```python
from build123d import *

# Parameters (mm, degrees)
CHAMFER1_SIZE          = 0.5
TROU_TARAUD_M30_REACH  = 42.606
TROU_TARAUD_M30_BORE_R = 1.25
CIRPATTERN1_COUNT      = 2
CIRPATTERN1_ANGLE      = 90


with BuildPart() as part:
    # Sketch1 → Revolve1 (revolve)
    with BuildSketch(Plane.XY, mode=Mode.PRIVATE) as revolve1_sk:
        Polygon((-7.15, 4), (-7.15, 14.67), (-6.65, 14.67), (-7.15, 19), (-6.15, 19), (-5, 16.17), (5, 16.17), (6.15, 19), (7.15, 19), (6.65, 14.67), (7.15, 14.67), (7.15, 11.75), (14.85, 11.75), (14.85, 4), align=None)
    revolve(revolve1_sk.sketch.rotate(Axis((0, 0, 0), (1, 0, 0)), 90), axis=Axis((0, 0, 0), (1, 0, 0)))

    # Chamfer1
    chamfer1_edges = [part.edges().sort_by_distance(p)[0] for p in [
        (14.85, 0, -11.75),
    ]]
    chamfer(chamfer1_edges, length=CHAMFER1_SIZE)

    # Trou taraudé M30 bore (on position points) → Trou taraudé M30 (cut, up to next)
    with BuildSketch(Plane(origin=(11.35, 0, 11.75), x_dir=(1, 0, 0), z_dir=(0, 0, 1)), mode=Mode.PRIVATE) as trou_taraud_m30_sk1:
        Circle(TROU_TARAUD_M30_BORE_R)
    trou_taraud_m30_tool1 = extrude(trou_taraud_m30_sk1.sketch, amount=-TROU_TARAUD_M30_REACH, mode=Mode.PRIVATE) & part.part
    trou_taraud_m30 = trou_taraud_m30_tool1.solids().sort_by_distance((11.35, 0, 11.75))[0]
    add(trou_taraud_m30, mode=Mode.SUBTRACT)

    # CirPattern1: Trou taraudé M30 ×2 about axis
    cirpattern1_axis = Axis((7.15, 0, 0), (-1, 0, 0))
    for i in range(1, CIRPATTERN1_COUNT):
        add(trou_taraud_m30.rotate(cirpattern1_axis, i * CIRPATTERN1_ANGLE / (CIRPATTERN1_COUNT - 1)), mode=Mode.SUBTRACT)


solid = part.part
```
Work out the finished part from the listing and answer in its coordinate system (mm). A direction names the side the tool comes from. Round coordinates to 2 decimals unless told otherwise and drop trailing zeros. Loops run counter-clockwise (first coordinate to the right, second up) from the corner with the lowest first, then second, coordinate; pieces in that order, holes last.
(1) Find the intervals of material crossed by L1, parallel to Z at x = 8, y = 0; L2, parallel to Y at x = -4.25, z = 0; L3, parallel to Z at x = 12, y = -3.5, in increasing order.
Computed values:
L1: z = -11.75 to -4, 4 to 11.75
L2: y = -16.17 to -4, 4 to 16.17
L3: z = -11.22 to -1.94, 1.94 to 11.22
(2) The part is cut by section D-D, the plane x = -5.5. Give the vertices of the cut face in (y, z).
Computed values:
outline: circle Ø34.8 at (0, 0); hole circle Ø8 at (0, 0)
(3) The part is cut by section C-C, the plane x = 2.5. Give the vertices of the cut face in (y, z).
Computed values:
outline: circle Ø32.34 at (0, 0); hole circle Ø8 at (0, 0)
(4) For faces 5 (the cylindrical face through (0.07, 15.785, -3.505)), 6 (the flat face through (-7.15, 3, -3)), 7 (the flat face through (7.15, -12, 0)), determine the directions among +Z, -Z, +X, -X, +Y, -Y from which every point of the face is accessible in a straight line to the end or side of a thin tool.
Computed values:
face 5: none
face 6: +Z, -Z, -X, +Y, -Y
face 7: +X
(5) Each of these flat-tipped pins is pushed along its axis until it touches: P1, Ø1, axis at x = 1, y = -13, coming from the +Z side; P2, Ø1.5, axis at x = 1, y = -3, coming from the +Z side; P3, Ø1.5, axis at y = -11.5, z = -7, coming from the +X side. Where does it stop, or does it pass through?
Computed values:
P1: stops at z = 10.26
P2: stops at z = 16.01
P3: stops at x = 7.15
(6) The part is cut by section A-A, the plane z = 0. Give the number of separate pieces and of enclosed holes in the cut face, and give its area (3 significant figures).
Computed values:
separate pieces: 3
enclosed holes: 0
area: 461 mm2
(7) The mould has two halves that part along Y. Classify faces 1 (the cylindrical face through (10.1, 7.83, -0.05)), 2 (the cylindrical face through (-6.643, 18.548, -4.119)), 3 (the cylindrical face through (10.1, 0.05, 7.83)), 4 (the cylindrical face through (6.9, 8.93, -11.64)): pulls with the +Y half, pulls with the -Y half, needs draft (parallel to the pull), parting line crosses it, or undercut.
Computed values:
face 1: needs draft
face 2: parting line crosses it
face 3: undercut
face 4: undercut
